Part model, mm, in its own coordinate system. A direction names the side the tool comes from. Coordinates: 2 decimals unless noted, no trailing zeros. Write each loop counter-clockwise with the first axis right and the second up, starting at its lowest first coordinate (ties: lowest second). Pieces come first, ordered by that corner, then holes. Notation, with made-up numbers: (-20, -23) -> (15, -23) arc R13 cw to (15, 0) -> close; hole circle Ø6 at (34.5, -30.75). An arc over 180 degrees is marked (long way). Write item = value, one per line.
from build123d import *

# Parameters (mm, degrees)
SKETCH1_W                = 2.54
SKETCH1_H                = 2.54
BOSS_EXTRUDE1_DEPTH      = 2.54
SKETCH2_W                = 0.65
SKETCH2_H                = 0.65
BOSS_EXTRUDE2_DEPTH      = 5.7
BOSS_EXTRUDE2_DEPTH_BACK = 5.64
CHAMFER1_SIZE            = 0.3
CHAMFER1_SIZE2           = 0.091719204
CHAMFER1_PART_2_SIZE     = 0.3
CHAMFER1_PART_2_SIZE2    = 0.091719204
CHAMFER1_PART_3_SIZE     = 0.3
CHAMFER1_PART_3_SIZE2    = 0.091719204
CHAMFER1_PART_4_SIZE     = 0.3
CHAMFER1_PART_4_SIZE2    = 0.091719204
CHAMFER1_PART_5_SIZE     = 0.3
CHAMFER1_PART_5_SIZE2    = 0.091719204
CHAMFER3_SIZE            = 0.7
CHAMFER3_SIZE2           = 0.341412812
CHAMFER4_SIZE            = 0.7
CHAMFER4_SIZE2           = 0.341412812


with BuildPart() as part:
    # Sketch1 → Boss-Extrude1 (new body)
    with BuildSketch(Plane(origin=(0, 0, 0), x_dir=(1, 0, 0), z_dir=(0, 1, 0))):
        Rectangle(SKETCH1_W, SKETCH1_H)
    extrude(amount=BOSS_EXTRUDE1_DEPTH)

    # Sketch2 → Boss-Extrude2 (add, two sides)
    with BuildSketch(Plane(origin=(0, 2.54, 0), x_dir=(1, 0, 0), z_dir=(0, 1, 0))) as boss_extrude2_sk:
        Rectangle(SKETCH2_W, SKETCH2_H)
    extrude(amount=BOSS_EXTRUDE2_DEPTH)
    extrude(boss_extrude2_sk.sketch, amount=-BOSS_EXTRUDE2_DEPTH_BACK)

    # Chamfer1
    chamfer1_edges = [part.edges().sort_by_distance(p)[0] for p in [
        (-0.325, -3.1, 0),
        (0, -3.1, -0.325),
        (0.325, -3.1, 0),
        (0, -3.1, 0.325),
    ]]
    chamfer1_side = [part.faces().sort_by_distance(p)[0] for p in [
        (0, -3.1, 0),
    ]]
    chamfer(chamfer1_edges, length=CHAMFER1_SIZE, length2=CHAMFER1_SIZE2, reference=chamfer1_side[0])

    # Chamfer1 part 2
    chamfer1_part_2_edges = [part.edges().sort_by_distance(p)[0] for p in [
        (-0.325, 8.24, 0),
    ]]
    chamfer1_part_2_side = [part.faces().sort_by_distance(p)[0] for p in [
        (-0.325, 5.39, 0),
    ]]
    chamfer(chamfer1_part_2_edges, length=CHAMFER1_PART_2_SIZE, length2=CHAMFER1_PART_2_SIZE2, reference=chamfer1_part_2_side[0])

    # Chamfer1 part 3
    chamfer1_part_3_edges = [part.edges().sort_by_distance(p)[0] for p in [
        (0, 8.24, 0.325),
    ]]
    chamfer1_part_3_side = [part.faces().sort_by_distance(p)[0] for p in [
        (0, 5.39, 0.325),
    ]]
    chamfer(chamfer1_part_3_edges, length=CHAMFER1_PART_3_SIZE, length2=CHAMFER1_PART_3_SIZE2, reference=chamfer1_part_3_side[0])

    # Chamfer1 part 4
    chamfer1_part_4_edges = [part.edges().sort_by_distance(p)[0] for p in [
        (0.325, 8.24, 0),
    ]]
    chamfer1_part_4_side = [part.faces().sort_by_distance(p)[0] for p in [
        (0.325, 5.39, 0),
    ]]
    chamfer(chamfer1_part_4_edges, length=CHAMFER1_PART_4_SIZE, length2=CHAMFER1_PART_4_SIZE2, reference=chamfer1_part_4_side[0])

    # Chamfer1 part 5
    chamfer1_part_5_edges = [part.edges().sort_by_distance(p)[0] for p in [
        (0, 8.24, -0.325),
    ]]
    chamfer1_part_5_side = [part.faces().sort_by_distance(p)[0] for p in [
        (0, 5.39, -0.325),
    ]]
    chamfer(chamfer1_part_5_edges, length=CHAMFER1_PART_5_SIZE, length2=CHAMFER1_PART_5_SIZE2, reference=chamfer1_part_5_side[0])

    # Chamfer3
    chamfer3_edges = [part.edges().sort_by_distance(p)[0] for p in [
        (1.27, 2.54, 0),
        (1.27, 1.27, 1.27),
        (1.27, 1.27, -1.27),
    ]]
    chamfer3_side = [part.faces().sort_by_distance(p)[0] for p in [
        (1.27, 1.27, 0),
    ]]
    chamfer(chamfer3_edges, length=CHAMFER3_SIZE, length2=CHAMFER3_SIZE2, reference=chamfer3_side[0])

    # Chamfer4
    chamfer4_edges = [part.edges().sort_by_distance(p)[0] for p in [
        (-1.27, 2.54, 0),
        (-1.27, 1.27, 1.27),
        (-1.27, 1.27, -1.27),
    ]]
    chamfer4_side = [part.faces().sort_by_distance(p)[0] for p in [
        (-1.27, 1.27, 0),
    ]]
    chamfer(chamfer4_edges, length=CHAMFER4_SIZE, length2=CHAMFER4_SIZE2, reference=chamfer4_side[0])


solid = part.part
Q1. Saw through at C-C on z = 0.8. Give the cut face in (x, y), and give its area (3 significant figures).
Model answer:
outline = (-1.16, 0) -> (1.16, 0) -> (1.16, 2.07) -> (0.93, 2.54) -> (-0.93, 2.54) -> (-1.16, 2.07) -> close
area = 5.77 mm²
Q2. Probe line 1 (Y direction, x = -0.5, z = 0.35); line 2 (Z direction, x = -0.1, y = 6.5) (3 decimals). List the from-to ranges inside material, lowest first. Write a range as from..to.
Model answer:
line_1 = 0..2.54
line_2 = -0.325..0.325
Q3. Pin check, flat tips, straight feed: pin 1 (0.8 mm diameter, centred on x = -0.5, z = 0.5, fed in from -Y); pin 2 (0.5 mm diameter, centred on x = 0, y = -1, fed in from -Z) (3 decimals); pin 3 (1.5 mm diameter, centred on x = 0, y = 5.5, fed in from +Z) (3 decimals); pin 4 (1.5 mm diameter, centred on x = 0.5, z = 0.5, fed in from +Y). Stop position of each tip, or through.
Model answer:
pin_1 = -3.04
pin_2 = -0.325
pin_3 = 0.325
pin_4 = 8.24
Q4. Saw through at D-D on y = 3. Give the cut face in (x, z) (3 decimals).
Model answer:
outline = (-0.325, -0.325) -> (0.325, -0.325) -> (0.325, 0.325) -> (-0.325, 0.325) -> close
Q5. Saw through at A-A on y = 1.25. Give the cut face in (x, z).
Model answer:
outline = (-1.27, -0.57) -> (-0.93, -1.27) -> (0.93, -1.27) -> (1.27, -0.57) -> (1.27, 0.57) -> (0.93, 1.27) -> (-0.93, 1.27) -> (-1.27, 0.57) -> close
Q6. Saw through at B-B on x = -0.8. Give the cut face in (y, z).
Model answer:
outline = (0, -1.27) -> (2.54, -1.27) -> (2.54, 1.27) -> (0, 1.27) -> close
Q7. Which spindle directions (+Z, -Z, +X, -X, +Y, -Y) get a long thin tool onto all of the face, cutting with end or side? Do faces 1 (the face through (1, 0, 0)), 2 (the face through (1.27, 1, 0)). Say none if no direction does.
Model answer:
face_1 = -Y
face_2 = +Z, -Z, +X, +Y, -Y
